Can you work these out from the model? Positions are in its coordinate system, mm. Face numbers are marked on the shaded views. Give positions to 0.01 mm unless a question says otherwise; leave off trailing zeros. Loops run counter-clockwise (first coordinate to the right, second up) from the corner with the lowest first, then second, coordinate; pieces in that order, holes last. Notation, with made-up numbers: (-16.75, 41) -> (23.25, 41) arc R18 ccw to (23.25, 55) -> close; hole circle Ø4 at (-23, 50.25). An arc over 180 degrees is marked (long way). Return JSON: item names as keys, results as strings. Group by question number.
Q1. Suppose I cut it at A-A, the plane z = -16. Please give me the cut outline in (x, y).
Q2. I need wall thicknesses on line 1 along Y through (x, z) = (17, -9); line 2 along Z through (x, y) = (26, 11.5); line 3 along Z through (x, y) = (41, 10). Which ranges of each line are inside material? Lowest first, please. Write a range as [from, to].
Q3. Suppose I cut it at B-B, the plane x = 14. Please give me the cut outline in (y, z).
Q4. Thinking about a two-plate mould opening in X: for the marked faces 1, 2 and 3, which applies, pulls with the +X half, pulls with the -X half, needs draft (parallel to the pull), parting line crosses it, or undercut?
Q5. Will this pin go through, and if not, where does the flat tip stop? pin 1 (8 mm diameter, centred on x = 23, z = -15.5, fed in from +Y).
```python
from build123d import *

# Parameters (mm, degrees)
CROQUIS1_W              = 43
CROQUIS1_H              = 43
SALIENTE_EXTRUIR1_DEPTH = 11.9
CROQUIS2_W              = 27
CROQUIS2_H              = 27
CORTAR_EXTRUIR1_DEPTH   = 0.5
REDONDEO1_R             = 5


with BuildPart() as part:
    # Croquis1 → Saliente-Extruir1 (new body)
    with BuildSketch(Plane(origin=(0, 0, 0), x_dir=(1, 0, 0), z_dir=(0, 1, 0))):
        with Locations((21.5, 21.5)):
            Rectangle(CROQUIS1_W, CROQUIS1_H)
    extrude(amount=SALIENTE_EXTRUIR1_DEPTH)

    # Croquis2 → Cortar-Extruir1 (cut)
    with BuildSketch(Plane(origin=(0, 11.9, 0), x_dir=(1, 0, 0), z_dir=(0, 1, 0))):
        with Locations((21.5, 21.5)):
            Rectangle(CROQUIS2_W, CROQUIS2_H)
    extrude(amount=-CORTAR_EXTRUIR1_DEPTH, mode=Mode.SUBTRACT)

    # Redondeo1
    redondeo1_edges = [part.edges().sort_by_distance(p)[0] for p in [
        (0, 5.95, -43),
        (43, 5.95, -43),
        (43, 5.95, 0),
        (0, 5.95, 0),
    ]]
    fillet(redondeo1_edges, radius=REDONDEO1_R)


solid = part.part
```
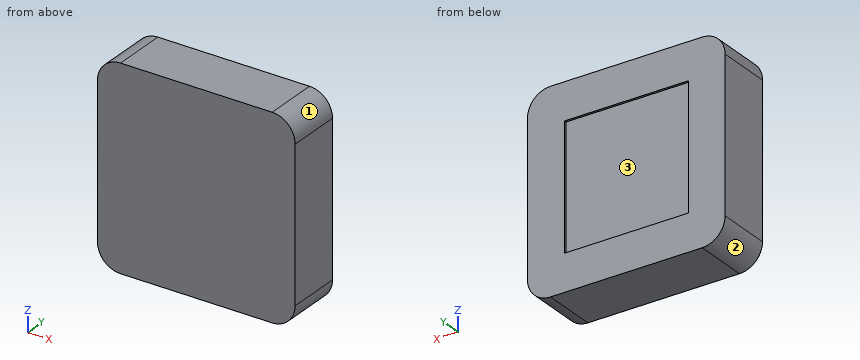
Ans:
{
 "1": {"outline": "(0, 0) -> (43, 0) -> (43, 11.9) -> (35, 11.9) -> (35, 11.4) -> (8, 11.4) -> (8, 11.9) -> (0, 11.9) -> close"},
 "2": {"line 1": "y = [0, 11.4]", "line 2": "z = [-43, -35], [-8, 0]", "line 3": "z = [-42, -1]"},
 "3": {"outline": "(0, -43) -> (11.9, -43) -> (11.9, -35) -> (11.4, -35) -> (11.4, -8) -> (11.9, -8) -> (11.9, 0) -> (0, 0) -> close"},
 "4": {"face 1": "pulls with the +X half", "face 2": "pulls with the -X half", "face 3": "undercut"},
 "5": {"pin 1": "stops at y = 11.4"}
}
